```python
from build123d import *

# Parameters (mm, degrees)
SKETCH1_W                = 20
SKETCH1_H                = 53
SKETCH1_R                = 2.5
BOSS_EXTRUDE1_DEPTH      = 18
FILLET1_R                = 10
BOSS_EXTRUDE2_DEPTH      = 18
BOSS_EXTRUDE3_DEPTH      = 43
BOSS_EXTRUDE3_DEPTH_BACK = 25
SKETCH3_W                = 20
SKETCH3_H                = 5
RIB8_REACH               = 69.365
SKETCH6_WALL_W           = 170.699933848
SKETCH6_WALL_H           = 5
RIB9_REACH               = 69.365
SKETCH7_WALL_W           = 170.699933848
SKETCH7_WALL_H           = 5
CUT_EXTRUDE1_DEPTH       = 69.366658541
CUT_EXTRUDE1_DEPTH_BACK  = 69.366658541
SKETCH8_R                = 2.5
SKETCH8_R_2              = 7.5
FILLET3_R                = 10
FILLET4_R                = 2


with BuildPart() as part:
    # Sketch1 → Boss-Extrude1 (new body)
    with BuildSketch(Plane.XY):
        with Locations((0, 13.5)):
            Rectangle(SKETCH1_W, SKETCH1_H)
        with Locations((0, 30)):
            Circle(SKETCH1_R, mode=Mode.SUBTRACT)
    extrude(amount=BOSS_EXTRUDE1_DEPTH)

    # Fillet1
    fillet1_edges = [part.edges().sort_by_distance(p)[0] for p in [
        (-10, 40, 9),
        (10, 40, 9),
    ]]
    fillet(fillet1_edges, radius=FILLET1_R - 0.0001)  # a hair under: the kernel refuses the full size

    # Sketch2 → Boss-Extrude2 (add)
    with BuildSketch(Plane.XY):
        Polygon((-10, 21.641016151), (-35, -13), (-10, -13), align=None)
        Polygon((10, 21.641016151), (10, -13), (23, -13), align=None)
    extrude(amount=BOSS_EXTRUDE2_DEPTH)

    # Sketch3 → Boss-Extrude3 (add, two sides: drawn at the far end of the back side and taken through both)
    with BuildSketch(Plane.XY.offset(-BOSS_EXTRUDE3_DEPTH_BACK)):
        with Locations((0, -10.5)):
            Rectangle(SKETCH3_W, SKETCH3_H)
    extrude(amount=BOSS_EXTRUDE3_DEPTH + BOSS_EXTRUDE3_DEPTH_BACK)

    # Sketch6 wall → Rib8 (add, up to next)
    with BuildSketch(Plane(origin=(-10, 3.5, -12.5), x_dir=(0, 0.677056530821, 0.735931011762), z_dir=(0, 0.735931011762, -0.677056530821)), mode=Mode.PRIVATE) as rib8_sk1:
        with Locations((0, 2.5)):
            Rectangle(SKETCH6_WALL_W, SKETCH6_WALL_H)
    rib8_tool1 = extrude(rib8_sk1.sketch, amount=-RIB8_REACH, mode=Mode.PRIVATE) - part.part
    rib8 = rib8_tool1.solids().sort_by_distance((-10, 3.5, -12.5))[0]
    add(rib8)

    # Sketch7 wall → Rib9 (add, up to next)
    with BuildSketch(Plane(origin=(-10, 3.5, 30.5), x_dir=(0, -0.677056530821, 0.735931011762), z_dir=(0, 0.735931011762, 0.677056530821)), mode=Mode.PRIVATE) as rib9_sk1:
        with Locations((0, 2.5)):
            Rectangle(SKETCH7_WALL_W, SKETCH7_WALL_H)
    rib9_tool1 = extrude(rib9_sk1.sketch, amount=-RIB9_REACH, mode=Mode.PRIVATE) - part.part
    rib9 = rib9_tool1.solids().sort_by_distance((-10, 3.5, 30.5))[0]
    add(rib9)

    # Mirror1: Rib8, Rib9 across plane
    add(rib8.mirror(Plane(origin=(0, 0, 0), x_dir=(0, 0, 1), z_dir=(1, 0, 0))))
    add(rib9.mirror(Plane(origin=(0, 0, 0), x_dir=(0, 0, 1), z_dir=(1, 0, 0))))

    # Sketch8 → Cut-Extrude1 (cut, two sides: drawn at the far end of the back side and taken through both)
    with BuildSketch(Plane(origin=(0, 0, 0), x_dir=(1, 0, 0), z_dir=(0, 1, 0)).offset(-CUT_EXTRUDE1_DEPTH_BACK)):
        with Locations(Location((0, 20, 0), (0, 0, 270))):
            Circle(SKETCH8_R)
        with Locations(Location((0, -38, 0), (0, 0, 270))):
            Circle(SKETCH8_R)
        with Locations(Location((-22.5, -9, 0), (0, 0, 270))):
            Circle(SKETCH8_R_2)
    extrude(amount=CUT_EXTRUDE1_DEPTH + CUT_EXTRUDE1_DEPTH_BACK, mode=Mode.SUBTRACT)

    # Fillet3
    fillet3_edges = [part.edges().sort_by_distance(p)[0] for p in [
        (-10, 21.641016151, 9),
        (10, 21.641016151, 9),
    ]]
    fillet(fillet3_edges, radius=FILLET3_R)

    # Fillet4
    fillet4_edges = [part.edges().sort_by_distance(p)[0] for p in [
        (-5, 3.5, 18),
        (-7.5, 15, 18),
        (0, -8, 0),
        (7.5, 15, 0),
        (5, 3.5, 0),
        (0, -8, 18),
        (5, 3.5, 18),
        (7.5, 15, 18),
        (-7.5, 15, 0),
        (-5, 3.5, 0),
    ]]
    fillet(fillet4_edges, radius=FILLET4_R)


solid = part.part
```
Could you check a few things on this model? Use its own coordinates, in mm. A direction names the side the tool comes from. Coordinates: 2 decimals unless noted, no trailing zeros. Write each loop counter-clockwise with the first axis right and the second up, starting at its lowest first coordinate (ties: lowest second). Pieces come first, ordered by that corner, then holes. Notation, with made-up numbers: (54.25, 16) -> (108.25, 16) arc R23 ccw to (108.25, 40) -> close; hole circle Ø4 at (53.5, -1.75). An arc over 180 degrees is marked (long way). Write item = value, one per line. Start each with the question number.
(1) I need wall thicknesses on line 1 (Z direction, x = 0, y = -11); line 2 (Y direction, x = 0, z = 5); line 3 (X direction, y = -7, z = 32.5). Which ranges of each line are inside material? Lowest first, please. Write a range as [from, to].
(2) I want a section at C-C (x = -20). Please give me the cut outline in (y, z).
(3) Will these pins go through, and if not, where does the flat tip stop? pin 1 (6.5 mm diameter, centred on x = 0, y = 30, fed in from -Z); pin 2 (8 mm diameter, centred on y = 5.5, z = 3.5, fed in from +X); pin 3 (16 mm diameter, centred on x = -8, y = 9.5, fed in from -Z); pin 4 (13.5 mm diameter, centred on x = -22.5, z = 9, fed in from -Y).
(4) I want a section at A-A (z = 12). Give the number of separate pieces and of enclosed holes in the cut face, plus the area to 3 significant figures.
(5) We'd pull the mould along X, two halves only. Please class faces 1 (the face through (-10, -3, 26)), 2 (the face through (10.165, 21.645, 9.126)), 3 (the face through (-5, -2, 27)): released by +X, released by -X, zero draft, split by the parting line, or undercut.
(6) I want a section at B-B (z = 38). Please give me the cut outline in (x, y), plus the area to 3 significant figures.
(7) I want a section at D-D (z = -9). Please give me the cut outline in (x, y), plus the area to 3 significant figures.
(8) Which directions (+Z, -Z, +X, -X, +Y, -Y) give clear straight access to the entire face, cutting with the end or side of a thin tool? Please do faces 4 (the face through (10, 27, 9)), 5 (the face through (-4.4, 4.11, -0.57)), 6 (the face through (-10, 27, 9)).
Result set:
q1.line_1 = [-25, -22.5], [-17.5, 35.5], [40.5, 43]
q1.line_2 = [-13, 27.5], [32.5, 40]
q1.line_3 = [-10, -5], [5, 10]
q2.outline = (-13, 0) -> (7.78, 0) -> (7.78, 1.93) -> (-13, 1.93) -> close; (-13, 16.07) -> (7.78, 16.07) -> (7.78, 18) -> (-13, 18) -> close
q3.pin_1 = 0
q3.pin_2 = 17.56
q3.pin_3 = -14.67
q3.pin_4 = through
q4.separate_pieces = 2
q4.enclosed_holes = 1
q4.area = 1,420 mm2
q5.face_1 = released by -X
q5.face_2 = released by +X
q5.face_3 = undercut
q6.outline = (-10, -13) -> (-2.5, -13) -> (-2.5, -8) -> (-5, -8) -> (-5, -3.4) -> (-10, -3.4) -> close; (2.5, -13) -> (10, -13) -> (10, -3.4) -> (5, -3.4) -> (5, -8) -> (2.5, -8) -> close
q6.area = 121 mm2
q7.outline = (-10, -13) -> (10, -13) -> (10, 6.72) -> (5, 6.72) -> (5, -8) -> (-5, -8) -> (-5, 6.72) -> (-10, 6.72) -> close
q7.area = 247 mm2
q8.face_4 = +Z, -Z, +X, +Y
q8.face_5 = -Z, +Y
q8.face_6 = +Z, -Z, -X, +Y
